Design review of the part built by this model. Coordinates are the model's own, in mm. Face numbers are marked on the shaded views. Round coordinates to 2 decimals unless told otherwise and drop trailing zeros. Loops run counter-clockwise (first coordinate to the right, second up) from the corner with the lowest first, then second, coordinate; pieces in that order, holes last. Notation, with made-up numbers: (-0.5, 10.25) -> (25.5, 10.25) arc R14 ccw to (25.5, 23.25) -> close; hole circle Ø10 at (-0.75, 31). An arc over 180 degrees is marked (long way). Write each question's results on one line, items separated by ' | '. Start each with the question number.
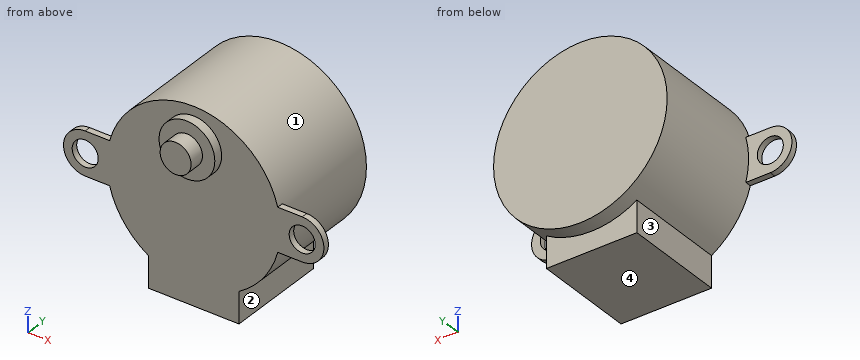
from build123d import *

# Parameters (mm, degrees)
CYLINDER004_R     = 2.5
CYLINDER004_DEPTH = 2.5
CYLINDER003_R     = 14
CYLINDER003_DEPTH = 19
SKETCH_R          = 2.1
EXTRUDE002_DEPTH  = 1
BOX003_W          = 14.6
BOX003_H          = 16.5
BOX003_DEPTH      = 17
CYLINDER002_R     = 4.5
CYLINDER002_DEPTH = 1.5


with BuildPart() as motor_shaft_part:
    # Cylinder004 → Cylinder004 (new body)
    with BuildSketch(Plane(origin=(0, -4, 8), x_dir=(1, 0, 0), z_dir=(0, 1, 0))):
        Circle(CYLINDER004_R)
    extrude(amount=CYLINDER004_DEPTH)


with BuildPart() as motor_body:
    # Cylinder003 → Cylinder003 (new body)
    with BuildSketch(Plane(origin=(0, 0, 0), x_dir=(1, 0, 0), z_dir=(0, 1, 0))):
        Circle(CYLINDER003_R)
    extrude(amount=CYLINDER003_DEPTH)


with BuildPart() as motor_bracket:
    # Sketch → Extrude002 (new body)
    with BuildSketch(Plane.XZ):
        with BuildLine():
            ThreePointArc((-17.500018, 3.5), (-21, -1.8e-05), (-17.499982, -3.5))
            Line((-17.499982, -3.5), (17.5, -3.5))
            ThreePointArc((17.5, -3.5), (21, 0), (17.5, 3.5))
            Line((-17.500018, 3.5), (17.5, 3.5))
        make_face()
        with Locations((17.5, 0)):
            Circle(SKETCH_R, mode=Mode.SUBTRACT)
        with Locations((-17.5, 0)):
            Circle(SKETCH_R, mode=Mode.SUBTRACT)
    extrude(amount=-EXTRUDE002_DEPTH)


with BuildPart() as motor_base:
    # Box003 → Box003 (new body)
    with BuildSketch(Plane(origin=(-7.3, 0, -17), x_dir=(1, 0, 0), z_dir=(0, 0, 1))):
        with Locations((7.3, 8.25)):
            Rectangle(BOX003_W, BOX003_H)
    extrude(amount=BOX003_DEPTH)


with BuildPart() as motor:
    # Cylinder002 → Cylinder002 (new body)
    with BuildSketch(Plane(origin=(0, -1.5, 8), x_dir=(1, 0, 0), z_dir=(0, 1, 0))):
        Circle(CYLINDER002_R)
    extrude(amount=CYLINDER002_DEPTH)

    # Fusion003: union motor_shaft_part, motor_body, motor_bracket, motor_base
    add(motor_shaft_part.part)
    add(motor_body.part)
    add(motor_bracket.part)
    add(motor_base.part)


with BuildPart() as motor_1:
    # Fusion003 placement: moved
    add(motor.part.moved(Location((0, 9, -8))))


solid = motor_1.part
1) Insertion check: pin 1 (5.5 mm diameter, centred on x = -3, z = -23.5, fed in from +Y); pin 2 (6 mm diameter, centred on x = 3, z = -21.5, fed in from -Y); pin 3 (0.5 mm diameter, centred on x = 14.5, y = 9.5, fed in from -Z); pin 4 (6.5 mm diameter, centred on x = -17.5, z = -8, fed in from +Y). Each pin has a flat end and moves straight along its axis. Give the tip position at first contact, or say it passes through.
2) Take a section at B-B (x = 0). Write out the cut boundary in (y, z), plus the area to 4 significant figures.
3) Take a section at C-C (x = -16). Write out the cut boundary in (y, z).
4) To check wall thickness, follow line 1 (Z direction, x = 17.5, y = 9.4); line 2 (Y direction, x = -2.5, z = -1); line 3 (Y direction, x = 5, z = -17.5). State the ranges of each line that lie inside material, in increasing order. Write a range as from..to.
5) Take a section at A-A (z = -8). Write out the cut boundary in (x, y).
6) The part is to be moulded in two halves that separate along X. For the marked faces 1, 2, 3 and 4, say which applies: +X half, -X half, draft (parallel to the pull), parting line (faces both ways), or undercut.
7) Take a section at D-D (z = 0.5). Write out the cut boundary in (x, y).
Geometry check:
1) pin 1: stops at y = 28 | pin 2: stops at y = 9 | pin 3: stops at z = -11.5 | pin 4: stops at y = 10
2) outline: (5, -2.5) -> (7.5, -2.5) -> (7.5, -4.5) -> (9, -4.5) -> (9, -25) -> (25.5, -25) -> (25.5, -22) -> (28, -22) -> (28, 6) -> (9, 6) -> (9, 4.5) -> (7.5, 4.5) -> (7.5, 2.5) -> (5, 2.5) -> close | area: 607.5 mm^2
3) outline: (9, -11.5) -> (10, -11.5) -> (10, -9.47) -> (9, -9.47) -> close; (9, -6.53) -> (10, -6.53) -> (10, -4.5) -> (9, -4.5) -> close
4) line 1: z = -11.5..-10.1, -5.9..-4.5 | line 2: y = 7.5..28 | line 3: y = 9..28
5) outline: (-21, 9) -> (-19.6, 9) -> (-19.6, 10) -> (-21, 10) -> close; (-15.4, 9) -> (15.4, 9) -> (15.4, 10) -> (14, 10) -> (14, 28) -> (-14, 28) -> (-14, 10) -> (-15.4, 10) -> close; (19.6, 9) -> (21, 9) -> (21, 10) -> (19.6, 10) -> close
6) face 1: parting line | face 2: +X half | face 3: -X half | face 4: draft
7) outline: (-11.12, 9) -> (-4.47, 9) -> (-4.47, 7.5) -> (-2.45, 7.5) -> (-2.45, 5) -> (2.45, 5) -> (2.45, 7.5) -> (4.47, 7.5) -> (4.47, 9) -> (11.12, 9) -> (11.12, 28) -> (-11.12, 28) -> close
